Autodesk Inventor part; units mm, degrees
ref_plane "Начальная плоскость" through (0, 0, 23) normal (0, 0, 1) x (1, 0, 0)
ref_plane "Конечная плоскость" through (0, 0, 627) normal (0, 0, 1) x (1, 0, 0)
ref_plane "РабПлоскость8" through (-227, -50, 23) normal (0, 0, -1) x (-1, 0, 0)
ref_plane "Начальная плоскость" through (0, 0, 23) normal (0, 0, 1) x (1, 0, 0)
ref_plane "Конечная плоскость" through (0, 0, 627) normal (0, 0, 1) x (1, 0, 0)
sketch "Эскиз" plane through (0, 0, 0) normal (0, 0, 1) x (1, 0, 0)
  line L0 (46, -50) -> (0, -50)
  line L1 (46, -50) -> (46, -46.6496)
  line L2 (43.2392, -43.6591) -> (10.9418, -41.0753)
  line L3 (4.5, -34.0976) -> (4.5, 34.0976)
  line L4 (43.2392, 43.6591) -> (10.9418, 41.0753)
  line L5 (46, 46.6496) -> (46, 50)
  line L6 (0, 50) -> (46, 50)
  line L7 (0, -50) -> (0, 50)
  arc A0 (4.5, -34.0976) -> (10.9418, -41.0753) centre (11.5, -34.0976) ccw
  arc A1 (10.9418, 41.0753) -> (4.5, 34.0976) centre (11.5, 34.0976) ccw
  arc A2 (46, -46.6496) -> (43.2392, -43.6591) centre (43, -46.6496) ccw
  arc A3 (43.2392, 43.6591) -> (46, 46.6496) centre (43, 46.6496) ccw
  line L8 (0, 70) -> (0, -70) construction
  line L9 (-9.3169, 0) -> (55.9016, 0) construction
  point P0 (46, -43.88)
  point P1 (4.5, -40.56)
  point P2 (4.5, 40.56)
  point P3 (46, 43.88)
  dimension "d3" = 46
  dimension "d5" = 4.5
  dimension "d7" = 100
  dimension "d9" = 9.44
  dimension "d11" = 9.44
  dimension "d13" = 6.12
  dimension "d15" = 6.12
  dimension "d22" = 7
  dimension "d23" = 3
  dimension "d24" = 50
  dimension "d25" = 0
extrude "Тело" add sketch "Эскиз" along normal up to surface (604 mm away) from surface at 23
sketch "Sketch3" plane through (0, 0, 0) normal (0, 0, 1) x (1, 0, 0)
  line L0 (0, 0) -> (10, 0)
ref_plane "Work Plane7" through (0, 0, 0) normal (0, -1, 0) x (1, 0, 0)
sketch "Sketch4" plane through (0, 0, 0) normal (0, -1, 0) x (1, 0, 0)
  line L0 (-2, 23) -> (12, 23)
  line L1 (-2, 627) -> (12, 627)
  dimension "d29" = 604
ref_plane "РабПлоскость8" through (-227, -50, 23) normal (0, 0, -1) x (-1, 0, 0)
split "Разделение1" plane through (-227, -50, 23) removes the side toward (0, 0, -1)
ref_plane "РабПлоскость9" through (23, -50, 627) normal (0, 0, 1) x (1, 0, 0)
split "Разделение2" plane through (23, -50, 627) removes the side toward (0, 0, 1)
equation "\"d3\" = b"
equation "\"d7\" = ParH"
equation "\"d22\" = R"
equation "\"d23\" = R1"
equation "\"d24\" = 0.5 * d7"
equation "\"d16\" = G_L"
equation "\"R1\" = 3"
equation "\"R\" = 7"
equation "\"t1\" = 4.5"
equation "\"t2\" = 7.6"
equation "\"ParH\" = 100"
equation "\"b\" = 46"
equation "\"msp_x1\" = 0.04 * b"
equation "\"msp_x2\" = -0.08 * t1 + 0.04 * b"
equation "\"G_L\" = d29"
equation "\"ex\" = 0"
equation "\"G_OFFSET_START\" = -23"
equation "\"G_OFFSET_END\" = -23"
equation "\"d26\" = -G_OFFSET_START"
equation "\"d27\" = G_OFFSET_END + B_L"
properties part number "Швеллер 10U-604 ГОСТ 8240-97" material "Сталь, мягкая, сварочная"
Here's how the part is built. I have some questions about the finished solid (model axes, mm). A direction names the side the tool comes from. Coordinates: 2 decimals unless noted, no trailing zeros. Write each loop counter-clockwise with the first axis right and the second up, starting at its lowest first coordinate (ties: lowest second). Pieces come first, ordered by that corner, then holes. Notation, with made-up numbers: (-28.5, 86) -> (22.5, 86) arc R20 ccw to (22.5, 116) -> close; hole circle Ø6 at (-14.75, 53). An arc over 180 degrees is marked (long way). Use a Markdown table: item, result. Add a question column.
(1) We'd pull the mould along Y, two halves only. Please class faces 3 (the flat face through (4, 4, 23)), 4 (the flat face through (23, -50, 321)), 5 (the flat face through (27.317, -42.385, 320.772)), 6 (the flat face through (23, 50, 321)): +Y half, -Y half, draft (parallel to the pull), parting line (faces both ways), or undercut.
(2) If we section it at C-C, the plane y = -22.5: Write out the boundary of the cut face in (x, z).
(3) For faces 1 (the flat face through (0, -1, 321)), 2 (the flat face through (4.5, 0, 321)), which set-ups out of +Z, -Z, +X, -X, +Y, -Y let a thin tool reach every point of the face, with its end or its side?
(4) If we section it at A-A, the plane x = 19: Write out the boundary of the cut face in (y, z).
(5) Please list where these lines run through material, in increasing order: line 1 (Y direction, x = 12, z = 518); line 2 (Y direction, x = 10.5, z = 508.5); line 3 (X direction, y = 26, z = 210).
(6) If we section it at B-B, the plane z = 306: Write out the boundary of the cut face in (x, y).
Outcome:
| question | item | result |
|---|---|---|
| 1 | face 3 | draft |
| 1 | face 4 | -Y half |
| 1 | face 5 | undercut |
| 1 | face 6 | +Y half |
| 2 | outline | (0, 23) -> (4.5, 23) -> (4.5, 627) -> (0, 627) -> close |
| 3 | face 1 | +Z, -Z, -X, +Y, -Y |
| 3 | face 2 | +Z, -Z, +X |
| 4 | outline | (-50, 23) -> (-41.72, 23) -> (-41.72, 627) -> (-50, 627) -> close; (41.72, 23) -> (50, 23) -> (50, 627) -> (41.72, 627) -> close |
| 5 | line 1 | y = -50 to -41.16, 41.16 to 50 |
| 5 | line 2 | y = -50 to -41.03, 41.03 to 50 |
| 5 | line 3 | x = 0 to 4.5 |
| 6 | outline | (0, -50) -> (46, -50) -> (46, -46.65) arc R3 ccw to (43.24, -43.66) -> (10.94, -41.08) arc R7 cw to (4.5, -34.1) -> (4.5, 34.1) arc R7 cw to (10.94, 41.08) -> (43.24, 43.66) arc R3 ccw to (46, 46.65) -> (46, 50) -> (0, 50) -> close |
